from build123d import *

# Parameters (mm, degrees)
F0_R         = 50
F1_DEPTH     = 15
F2_T         = -3
F4_DEPTH     = 20
F5_R         = 13
F6_DEPTH     = 35.001
F7_T         = 3
F7_T3_DEPTH  = 47.5692193817
F7_T5_DEPTH  = 47.5692193817
F7_T7_DEPTH  = 47.5692193817
F7_T10_ANGLE = 120.000000001
F7_T12_ANGLE = 120.000000001
F7_T14_ANGLE = 120.000000001
F8_R         = 3


# Not quite as in the source:
# - a shell that OpenCascade refuses in one call is made with other operations: the cavity is built on its own and cut out


with BuildPart() as f1:
    # F0 (on Top) → F1 (new body)
    with BuildSketch(Plane.XY):
        Circle(F0_R)
    extrude(amount=-F1_DEPTH)

    # F2
    f2_openings = [f1.faces().sort_by_distance(p)[0] for p in [
        (0, 0, -15),
    ]]
    offset(amount=F2_T, openings=f2_openings)

    # F3 (on face) → F4 (join)
    with BuildSketch(Plane.XY):
        with BuildLine():
            Line((36.3730669589, -3), (15.5884572681, 33))
            ThreePointArc((15.5884572681, 33), (0, 42), (-15.5884572681, 33))
            Line((-15.5884572681, 33), (-36.3730669589, -3))
            ThreePointArc((-36.3730669589, -3), (-36.3730669589, -21), (-20.7846096908, -30))
            Line((-20.7846096908, -30), (20.7846096908, -30))
            ThreePointArc((20.7846096908, -30), (36.3730669589, -21), (36.3730669589, -3))
        make_face()
    extrude(amount=F4_DEPTH)

    # F5 (on face) → F6 (cut, through all)
    with BuildSketch(Plane.XY.offset(20)):
        with Locations((0, 24)):
            Circle(F5_R)
        with Locations((-20.7846096908, -12)):
            Circle(F5_R)
        with Locations((20.7846096908, -12)):
            Circle(F5_R)
    extrude(amount=-F6_DEPTH, mode=Mode.SUBTRACT)

    # F7: shell of thickness 3, made by hand


with BuildPart() as f7_core1:
    # F7_t2: copy of F1
    add(f1.part)

    # the walls: a layer under each face that stays
    f7_faces = [f7_core1.faces().sort_by_distance(p)[0] for p in [
        (-50, 0, -7.5),
        (-33.3333333333, -33.3333333333, 0),
        (-33.3333333333, -33.3333333333, -15),
        (25.9807621135, 15, 10),
        (0, 42, 10),
        (-25.9807621135, 15, 10),
        (-36.3730669589, -21, 10),
        (0, -30, 10),
        (36.3730669589, -21, 10),
        (-47, 0, -9),
        (0, 0, -3),
        (-33.7846096908, -12, 8.5),
        (7.7846096908, -12, 8.5),
        (-13, 24, 8.5),
    ]]
    thicken(f7_faces, amount=-F7_T, mode=Mode.SUBTRACT)

    # F7_s4 → F7_t3 (cut)
    with BuildSketch(Plane(origin=(11.8923048454, -20.5980762114, 0), x_dir=(0, 0, 1), z_dir=(-0.5, 0.8660254038, 0))):
        Polygon((0.03, 30.03), (-3, 30), (-3, 27), (0, 27), align=None)
    extrude(amount=F7_T3_DEPTH, mode=Mode.SUBTRACT)

    # F7_s6 → F7_t5 (cut)
    with BuildSketch(Plane(origin=(11.8923048454, 20.5980762114, 0), x_dir=(0, 0, 1), z_dir=(-0.5, -0.8660254038, 0))):
        Polygon((0.03, 30.03), (-3, 30), (-3, 27), (0, 27), align=None)
    extrude(amount=F7_T5_DEPTH, mode=Mode.SUBTRACT)

    # F7_s8 → F7_t7 (cut)
    with BuildSketch(Plane.YZ.offset(-23.7846096908)):
        Polygon((-30.03, 0.03), (-30, -3), (-27, -3), (-27, 0), align=None)
    extrude(amount=F7_T7_DEPTH, mode=Mode.SUBTRACT)

    # F7_s9 → F7_t10 (revolve, cut)
    with BuildSketch(Plane(origin=(-10.3923048454, 18, 0), x_dir=(0, 0, 1), z_dir=(0.5, -0.8660254038, 0))):
        Polygon((0.03, -30.03), (-3, -30), (-3, -27), (0, -27), align=None)
    revolve(axis=Axis((0, 24, 0), (0, 0, 1)), revolution_arc=F7_T10_ANGLE, mode=Mode.SUBTRACT)

    # F7_s11 → F7_t12 (revolve, cut)
    with BuildSketch(Plane(origin=(-10.3923048454, -18, 0), x_dir=(0, 0, 1), z_dir=(0.5, 0.8660254038, 0))):
        Polygon((0.03, -30.03), (-3, -30), (-3, -27), (0, -27), align=None)
    revolve(axis=Axis((-20.7846096908, -12, 0), (0, 0, 1)), revolution_arc=F7_T12_ANGLE, mode=Mode.SUBTRACT)

    # F7_s13 → F7_t14 (revolve, cut)
    with BuildSketch(Plane.YZ.offset(20.7846096908)):
        Polygon((-30.03, 0.03), (-30, -3), (-27, -3), (-27, 0), align=None)
    revolve(axis=Axis((20.7846096908, -12, 0), (0, 0, 1)), revolution_arc=F7_T14_ANGLE, mode=Mode.SUBTRACT)

    # F7_s15 → F7_t16 (revolve, cut)
    with BuildSketch(Plane.XZ):
        Polygon((46.97, -3.03), (50, -3), (50, 0), (47, 0), align=None)
    revolve(axis=Axis((0, 0, -3), (0, 0, 1)), mode=Mode.SUBTRACT)


with BuildPart() as f1_1:
    add(f1.part)

    # what is left inside the walls is the cavity
    f7_cavity = [f7_core1.part.solids().sort_by_distance(p)[0] for p in [
        (6.902222, -3.985, 6.666667),
    ]]
    add(f7_cavity, mode=Mode.SUBTRACT)

    # F8
    f8_edges = [f1_1.edges().sort_by_distance(p)[0] for p in [
        (6.928203, -4, 0),
        (23.382686, 13.5, 0),
        (0, 8, 0),
        (-23.382686, 13.5, 0),
        (-6.928203, -4, 0),
        (0, -27, 0),
        (-25.980762, 15, 0),
        (-50, 0, 0),
        (25.980762, 15, 0),
        (0, 42, 0),
        (-36.373067, -21, 0),
        (0, -30, 0),
        (36.373067, -21, 0),
        (15.774263, 26.678175, 10),
        (30.991109, 0.321825, 10),
        (-15.774263, 26.678175, 10),
        (-30.991109, 0.321825, 10),
        (-15.216845, -27, 10),
        (15.216845, -27, 10),
    ]]
    fillet(f8_edges, radius=F8_R)


solid = f1_1.part
Could you check a few things on this model? Use its own coordinates, in mm. A direction names the side the tool comes from. Coordinates: 2 decimals unless noted, no trailing zeros. Order: outer loops, then holes, each group sorted by start corner. A loop starts at its lowest first (then second) coordinate and runs counter-clockwise, first axis right, second up.
Q1. Suppose I cut it at C-C on z = 9. Please give me the cut outline in (x, y).
Q2. Suppose I cut it at A-A on x = 0. Please give me the cut outline in (y, z), and give its area (3 significant figures).
Q3. Thinking about a two-plate mould opening in Y: for faces 5 (the cylindrical face through (0, 8, 12)), 6 (the cylindrical face through (47.69, 15.02, -8.92)), 7 (the flat face through (0, -30, 11)), which applies, released by +Y, released by -Y, zero draft, split by the parting line, or undercut?
Q4. Which directions (+Z, -Z, +X, -X, +Y, -Y) give clear straight access to the entire face, cutting with the end or side of a thin tool? Please do faces 1 (the cylindrical face through (-36.503, -20.771, 11.381)), 2 (the flat face through (-25.835, 15.252, 11.381)), 3 (the cylindrical face through (22.599, 13.146, 0.902)), 4 (the cylindrical face through (44.83, 14.12, -8.92)).
Q5. Will these pins go through, and if not, where does the flat tip stop? pin 1 (1.5 mm diameter, centred on y = 12, z = -6.5, fed in from -X); pin 2 (4 mm diameter, centred on y = -12.5, z = 13, fed in from -X); pin 3 (3 mm diameter, centred on x = 32.5, z = -1.5, fed in from +Y).
Q6. Suppose I cut it at D-D on y = -6.5. Give the number of separate pieces and of enclosed holes in the cut face, and give its area (3 significant figures).
Q7. Please list where these lines run through material, in increasing order: L1, parallel to Y at x = 0.5, z = 15; L2, parallel to Y at x = -24.5, z = 13; L3, parallel to Z at x = -7.5, y = -46.
Q8. Suppose I cut it at B-B on z = -11. Please give me the cut outline in (x, y), and give its area (3 significant figures).
Answer:
1. outline: (-36.37, -3) arc R18 ccw to (-20.78, -30) - (20.78, -30) arc R18 ccw to (36.37, -3) - (15.59, 33) arc R18 ccw to (-15.59, 33) - close; hole circle Ø26 at (-20.78, -12); hole (-26.41, 8.26) arc R3 ccw to (-23.33, 3.8) arc R16 cw to (-8.38, -22.11) arc R3 ccw to (-6.05, -27) - (6.05, -27) arc R3 ccw to (8.38, -22.11) arc R16 cw to (23.33, 3.8) arc R3 ccw to (26.41, 8.26) - (20.36, 18.74) arc R3 ccw to (14.95, 18.31) arc R16 cw to (-14.95, 18.31) arc R3 ccw to (-20.36, 18.74) - close; hole circle Ø26 at (0, 24); hole circle Ø26 at (20.78, -12)
2. outline: (-50, -15) - (-47, -15) - (-47, -3) - (11, -3) - (11, 20) - (8, 20) - (8, 3) arc R3 cw to (5, 0) - (-24, 0) arc R3 cw to (-27, 3) - (-27, 20) - (-30, 20) - (-30, 3) arc R3 cw to (-33, 0) - (-47, 0) arc R3 ccw to (-50, -3) - close; (37, -3) - (47, -3) - (47, -15) - (50, -15) - (50, -3) arc R3 ccw to (47, 0) - (45, 0) arc R3 cw to (42, 3) - (42, 20) - (37, 20) - close
2. area: 518 mm2
3. face 5: undercut
3. face 6: split by the parting line
3. face 7: released by -Y
4. face 1: +Z, -X
4. face 2: +Z, -X, +Y
4. face 3: +Z
4. face 4: -Z
5. pin 1: stops at x = -48.72
5. pin 2: stops at x = -38.78
5. pin 3: stops at y = 38.96
6. separate pieces: 3
6. enclosed holes: 0
6. area: 577 mm2
7. L1: y = -30 to -27, 8.01 to 11.01, 36.99 to 41.99
7. L2: y = -29.61 to -24.46, 0.46 to 3.84, 11.56 to 17.56
7. L3: z = -3 to 0
8. outline: circle Ø100 at (0, 0); hole circle Ø94 at (0, 0)
8. area: 914 mm2
